```python
from build123d import *

# Parameters (mm, degrees)
F0_W     = 113.869563
F0_H     = 83.149798
F1_DEPTH = 25.4
F2_R     = 22.535433
F3_DEPTH = 25.4
F5_DEPTH = 76.2


with BuildPart() as f1:
    # F0 (on Top) → F1 (new body)
    with BuildSketch(Plane.XY):
        with Locations((-56.934781, 41.574899)):
            Rectangle(F0_W, F0_H)
    extrude(amount=F1_DEPTH)

    # F2 (on face) → F3 (join)
    with BuildSketch(Plane.XY.offset(25.4)):
        with Locations((-59.87053, 41.805387)):
            Circle(F2_R)
    extrude(amount=F3_DEPTH)

    # F4 (on Front) → F5 (cut)
    with BuildSketch(Plane.XZ):
        Polygon((-102.13092, 49.10665), (-86.741515, 49.326494), (-31.999189, 30.639356), (-31.999189, 64.935751), align=None)
    extrude(amount=-F5_DEPTH, mode=Mode.SUBTRACT)


solid = f1.part
```
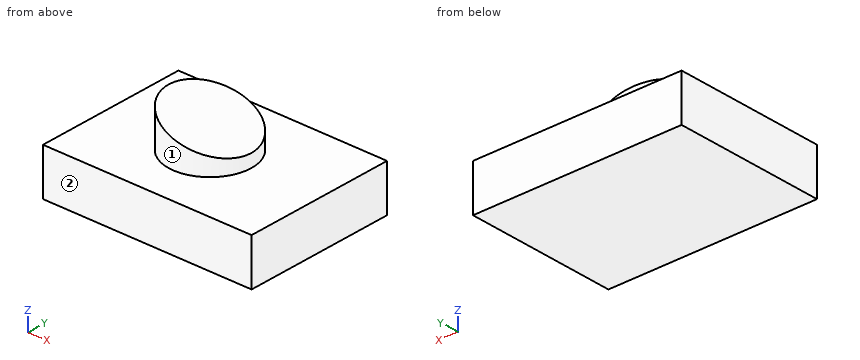
Part model, mm, in its own coordinate system. Face numbers are marked on the shaded views. A direction names the side the tool comes from. Coordinates: 2 decimals unless noted, no trailing zeros. Write each loop counter-clockwise with the first axis right and the second up, starting at its lowest first coordinate (ties: lowest second). Pieces come first, ordered by that corner, then holes.
Item 1: Which spindle directions (+Z, -Z, +X, -X, +Y, -Y) get a long thin tool onto all of the face, cutting with end or side? Do the marked faces 1 and 2. Say none if no direction does.
Item 2: Probe line 1 (Z direction, x = -39, y = 15); line 2 (Y direction, x = -60.5, z = 40); line 3 (Z direction, x = -66, y = 43.5). List the from-to ranges inside material, lowest first.
Item 3: Slice it at D-D (y = 38.5). Write the cut outline in (x, z).
Item 4: Slice it at A-A (y = 63). Write the cut outline in (x, z), and give its area (3 significant figures).
Item 5: Pin check, flat tips, straight feed: pin 1 (8 mm diameter, centred on y = 46.5, z = 33, fed in from -X); pin 2 (6 mm diameter, centred on x = -63, z = 15.5, fed in from -Y); pin 3 (12 mm diameter, centred on x = -48.5, y = 29.5, fed in from +Z); pin 4 (8 mm diameter, centred on y = 63.5, z = 41, fed in from -X). Stop position of each tip, or through.
Item 6: Slice it at C-C (z = 36.5). Write the cut outline in (x, y), and give its area (3 significant figures).
Item 7: Slice it at B-B (x = -10.5). Write the cut outline in (y, z), and give its area (3 significant figures).
Results found:
1. face 1: +Z
1. face 2: +Z, -Z, +X, -X, -Y
2. line 1: z = 0 to 25.4
2. line 2: y = 19.28 to 64.33
2. line 3: z = 0 to 42.25
3. outline: (-113.87, 0) - (0, 0) - (0, 25.4) - (-37.58, 25.4) - (-37.58, 32.54) - (-82.16, 47.76) - (-82.16, 25.4) - (-113.87, 25.4) - close
4. outline: (-113.87, 0) - (0, 0) - (0, 25.4) - (-52.21, 25.4) - (-52.21, 37.54) - (-67.53, 42.77) - (-67.53, 25.4) - (-113.87, 25.4) - close
4. area: 3,120 mm2
5. pin 1: stops at x = -82.4
5. pin 2: stops at y = 0
5. pin 3: stops at z = 38.32
5. pin 4: stops at x = -73.83
6. outline: (-49.17, 21.97) - (-49.17, 61.64) arc R22.54 ccw (long way) to start
6. area: 1,260 mm2
7. outline: (0, 0) - (83.15, 0) - (83.15, 25.4) - (0, 25.4) - close
7. area: 2,110 mm2
